Design review of the part shown in the three views and the two pictorial views. Dimensions are in mm from the part's minimum x, y and z. A direction names the side the tool comes from. Round coordinates to 2 decimals unless told otherwise and drop trailing zeros. Order: outer loops, then holes, each group sorted by start corner. A loop starts at its lowest first (then second) coordinate and runs counter-clockwise, first axis right, second up. Notation, with made-up numbers: (78.5, 62) - (105.5, 62) arc R34 cw to (105.5, 100) - close; hole circle Ø10 at (-23.5, 53.5). An arc over 180 degrees is marked (long way). One line per item, written item: value.
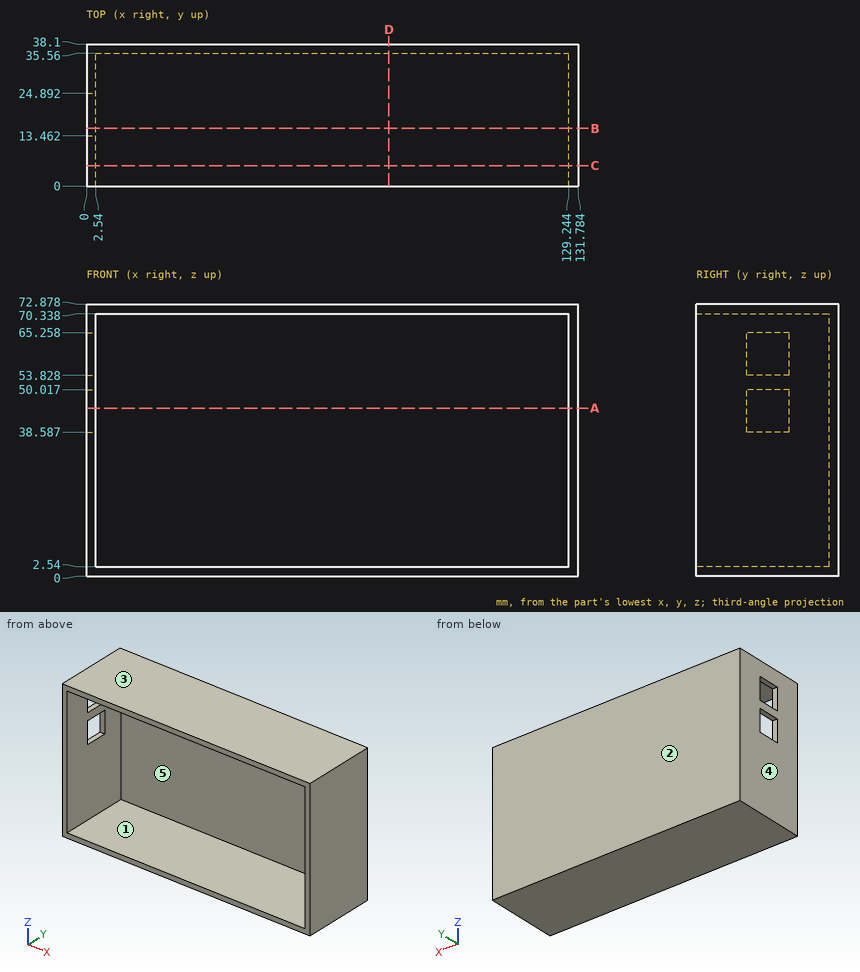
Item 1: Wall thickness on line 1 (Z direction, x = 85.5, y = 27.5); line 2 (X direction, y = 33, z = 28) (1 decimal); line 3 (Y direction, x = 88, z = 65): over which ranges is each line inside the solid? List them lowest first.
Returned:
line 1: 0 to 2.54, 70.34 to 72.88
line 2: 0 to 2.5, 129.2 to 131.8
line 3: 35.56 to 38.1
Item 2: The part is to be moulded in two halves that separate along X. For the marked faces 3, 4 and 5, say which applies: +X half, -X half, draft (parallel to the pull), parting line (faces both ways), or undercut.
Returned:
face 3: draft
face 4: -X half
face 5: undercut
Item 3: Take a section at C-C (y = 5.5). Write out the cut boundary in (x, z) (1 decimal), plus the area to 3 significant figures.
Returned:
outline: (0, 0) - (131.8, 0) - (131.8, 72.9) - (0, 72.9) - close; hole (2.5, 2.5) - (129.2, 2.5) - (129.2, 70.3) - (2.5, 70.3) - close
area: 1,010 mm^2
Item 4: Machinability: for the marked faces 1 and 2, which of the approach directions +Z, -Z, +X, -X, +Y, -Y give a long, thin tool a straight path to every point of the face, cutting with its end or side? Answer none if there is none.
Returned:
face 1: -Y
face 2: +Z, -Z, +X, -X, +Y
Item 5: Take a section at A-A (z = 45). Write out the cut boundary in (x, y) (1 decimal).
Returned:
outline: (0, 0) - (2.5, 0) - (2.5, 13.5) - (0, 13.5) - close; (0, 24.9) - (2.5, 24.9) - (2.5, 35.6) - (129.2, 35.6) - (129.2, 0) - (131.8, 0) - (131.8, 38.1) - (0, 38.1) - close
Item 6: For P1, Ø1.3, axis at x = 1.5, z = 42, coming from the -Y side; P2, Ø5, axis at x = 71, z = 55, coming from the -Y side, all flat-tipped, find the tip position at first contact; note any pin that passes through.
Returned:
P1: y = 0
P2: y = 35.56
Item 7: Take a section at B-B (y = 15.5). Write out the cut boundary in (x, z) (1 decimal).
Returned:
outline: (0, 0) - (131.8, 0) - (131.8, 72.9) - (0, 72.9) - (0, 65.3) - (2.5, 65.3) - (2.5, 70.3) - (129.2, 70.3) - (129.2, 2.5) - (2.5, 2.5) - (2.5, 38.6) - (0, 38.6) - close; (0, 50) - (2.5, 50) - (2.5, 53.8) - (0, 53.8) - close
Item 8: Take a section at D-D (x = 81). Write out the cut boundary in (y, z).
Returned:
outline: (0, 0) - (38.1, 0) - (38.1, 72.88) - (0, 72.88) - (0, 70.34) - (35.56, 70.34) - (35.56, 2.54) - (0, 2.54) - close
